Can you work these out from the model? Positions are in its coordinate system, mm. A direction names the side the tool comes from. Coordinates: 2 decimals unless noted, no trailing zeros. Order: outer loops, then holes, each group sorted by start corner. A loop starts at its lowest first (then second) coordinate and runs counter-clockwise, first axis right, second up. Notation, with made-up numbers: (0.25, -39.75) -> (21.25, -39.75) arc R6 cw to (21.25, -28.75) -> close; hole circle Ø9 at (51, -15.75). An arc over 180 degrees is marked (long way). Answer in a Markdown table with one row per item.
```python
from build123d import *

# Parameters (mm, degrees)
SKETCH1_R           = 0.9834
BOSS_EXTRUDE1_DEPTH = 8
SKETCH2_R           = 1.9334
BOSS_EXTRUDE2_DEPTH = 6
SKETCH3_R           = 3
BOSS_EXTRUDE3_DEPTH = 4
CUT_EXTRUDE1_DEPTH  = 2


with BuildPart() as part:
    # Sketch1 → Boss-Extrude1 (new body)
    with BuildSketch(Plane(origin=(0, 0, 0), x_dir=(0, 0, -1), z_dir=(1, 0, 0))):
        Circle(SKETCH1_R)
    extrude(amount=BOSS_EXTRUDE1_DEPTH)

    # Sketch2 → Boss-Extrude2 (add)
    with BuildSketch(Plane(origin=(8, 0, 0), x_dir=(0, 0, -1), z_dir=(1, 0, 0))):
        Circle(SKETCH2_R)
    extrude(amount=BOSS_EXTRUDE2_DEPTH)

    # Sketch3 → Boss-Extrude3 (add)
    with BuildSketch(Plane(origin=(14, 0, 0), x_dir=(0, 0, -1), z_dir=(1, 0, 0))):
        Circle(SKETCH3_R)
    extrude(amount=-BOSS_EXTRUDE3_DEPTH)

    # Sketch7 → Cut-Extrude1 (cut)
    with BuildSketch(Plane(origin=(14, 0, 0), x_dir=(0, 0, -1), z_dir=(1, 0, 0))):
        Polygon((2.040680279, 1.096176231), (0.071023676, 2.315369078), (-1.969656602, 1.219192847), (-2.040680279, -1.096176231), (-0.071023676, -2.315369078), (1.969656602, -1.219192847), align=None)
    extrude(amount=-CUT_EXTRUDE1_DEPTH, mode=Mode.SUBTRACT)


solid = part.part
```
(1) Suppose I cut it at A-A (y = 1.6). Please give me the cut outline in (x, z).
Response values:
| item | result |
|---|---|
| outline | (8, -1.09) -> (10, -1.09) -> (10, -2.54) -> (14, -2.54) -> (14, -1.23) -> (12, -1.23) -> (12, 1.26) -> (14, 1.26) -> (14, 2.54) -> (10, 2.54) -> (10, 1.09) -> (8, 1.09) -> close |
(2) Suppose I cut it at B-B (x = 3.5). Please give me the cut outline in (y, z).
Response values:
| item | result |
|---|---|
| outline | circle Ø1.97 at (0, 0) |
(3) We'd pull the mould along Z, two halves only. Please class faces 4 (the flat face through (10, -2, -1)), 5 (the cylindrical face through (3.94, -0.96, 0.21)), 6 (the flat face through (13.014, 1.697, -1.07)): +Z half, -Z half, draft (parallel to the pull), parting line (faces both ways), or undercut.
Response values:
| item | result |
|---|---|
| face 4 | draft |
| face 5 | parting line |
| face 6 | undercut |
(4) I need wall thicknesses on line 1 (X direction, y = 0.05, z = -2.35); line 2 (X direction, y = 0.55, z = -1.1); line 3 (Z direction, x = 13.75, y = -1). Which ranges of each line are inside material? Lowest first, please. Write a range as [from, to].
Response values:
| item | result |
|---|---|
| line 1 | [10, 14] |
| line 2 | [8, 12] |
| line 3 | [-2.83, -1.98], [2.04, 2.83] |
(5) On a 3-axis mill with a long thin cutter (end or side, diameter ignored), from which of +Z, -Z, +X, -X, +Y, -Y can I reach the whole of each face in a straight line? I mean faces 1 (the flat face through (8, -1, -1)), 2 (the flat face through (13.014, -1.775, -0.935)), 3 (the cylindrical face through (12, 0, 3)). Say none if no direction works.
Response values:
| item | result |
|---|---|
| face 1 | -X |
| face 2 | +X |
| face 3 | +X, -X |
(6) Suppose I cut it at C-C (z = -1.4). Please give me the cut outline in (x, y), and give its area (3 significant figures).
Response values:
| item | result |
|---|---|
| outline | (8, -1.33) -> (10, -1.33) -> (10, -2.65) -> (14, -2.65) -> (14, -1.53) -> (12, -1.53) -> (12, 1.49) -> (14, 1.49) -> (14, 2.65) -> (10, 2.65) -> (10, 1.33) -> (8, 1.33) -> close |
| area | 20.5 mm2 |
(7) Will these pins go through, and if not, where does the flat tip stop? pin 1 Ø1 at (x, y) = (3, -1) entering from +Z; pin 2 Ø1.2 at (y, z) = (-0.5, 1) entering from +X.
Response values:
| item | result |
|---|---|
| pin 1 | z = 0.85 |
| pin 2 | x = 12 |
(8) Suppose I cut it at D-D (y = -2.1). Please give me the cut outline in (x, z).
Response values:
| item | result |
|---|---|
| outline | (10, -2.14) -> (14, -2.14) -> (14, -0.33) -> (12, -0.33) -> (12, 0.42) -> (14, 0.42) -> (14, 2.14) -> (10, 2.14) -> close |
